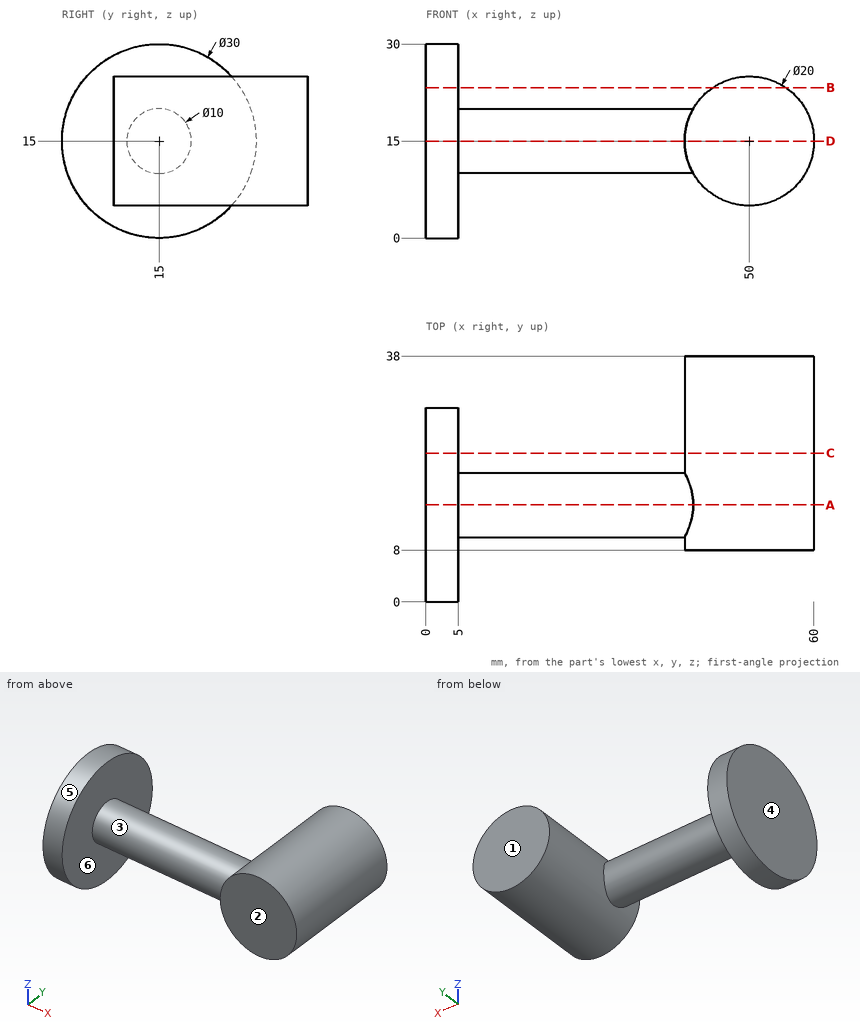
Verification items for this drawing (mm, ordinates from the low corner). A direction names the side the tool comes from. Round coordinates to 2 decimals unless told otherwise and drop trailing zeros. Loops run counter-clockwise (first coordinate to the right, second up) from the corner with the lowest first, then second, coordinate; pieces in that order, holes last. Notation, with made-up numbers: (21, 39) -> (70, 39) arc R12 ccw to (70, 62) -> close; hole circle Ø2 at (60.5, -9.75). An arc over 180 degrees is marked (long way). Write item = value, one per line. Start each with the question number.
1) Release check for a two-part mould opening along X. For the marked faces 4, 5 and 6 record: released by +X, released by -X, zero draft, split by the parting line, or undercut.
2) Sectioned sample at B-B, the plane z = 23.25. Record the cut outline in (x, y).
3) Sectioned sample at A-A, the plane y = 15. Record the cut outline in (x, z).
4) Sectioned sample at C-C, the plane y = 23. Record the cut outline in (x, z), plus the area to 3 significant figures.
5) Sectioned sample at D-D, the plane z = 15. Record the cut outline in (x, y).
6) Thickness scan on probe 1 along X at (y, z) = (20, 2.25); probe 2 along Y at (x, z) = (48, 19.75); probe 3 along X at (y, z) = (12.5, 9.25). Record the ranges inside material, lowest first.
7) Gauge pin test, flat ends, axial feed: pin 1 Ø6 at (y, z) = (23, 25) entering from +X; pin 2 Ø1 at (x, z) = (30, 11) entering from +Y; pin 3 Ø12 at (y, z) = (8.5, 11.5) entering from +X; pin 4 Ø6 at (x, z) = (54, 17) entering from -Y. Record the tip position at first contact, or that the pin passes through.
8) Set-up check for the marked faces 1, 2 and 3: record each of +Z, -Z, +X, -X, +Y, -Y from which the full face is reachable in a straight line by a thin tool's end or side.
Results are:
q1.face_4 = released by -X
q1.face_5 = zero draft
q1.face_6 = undercut
q2.outline = (0, 2.47) -> (5, 2.47) -> (5, 27.53) -> (0, 27.53) -> close; (44.35, 8) -> (55.65, 8) -> (55.65, 38) -> (44.35, 38) -> close
q3.outline = (0, 0) -> (5, 0) -> (5, 10) -> (41.34, 10) arc R10 ccw (long way) to (41.34, 20) -> (5, 20) -> (5, 30) -> (0, 30) -> close
q4.outline = (0, 2.31) -> (5, 2.31) -> (5, 27.69) -> (0, 27.69) -> close; circle Ø20 at (50, 15)
q4.area = 441 mm^2
q5.outline = (0, 0) -> (5, 0) -> (5, 10) -> (40, 10) -> (40, 8) -> (60, 8) -> (60, 38) -> (40, 38) -> (40, 20) -> (5, 20) -> (5, 30) -> (0, 30) -> close
q6.probe_1 = 0 to 5
q6.probe_2 = 8 to 38
q6.probe_3 = 0 to 5, 41.82 to 58.18
q7.pin_1 = 57.14
q7.pin_2 = 18.57
q7.pin_3 = 60
q7.pin_4 = 8
q8.face_1 = +Z, -Z, +X, -X, +Y
q8.face_2 = +Z, -Z, +X, -Y
q8.face_3 = none
